Geometry: final body of the model. Coordinates: model frame, mm. A direction names the side the tool comes from. Give positions to 0.01 mm unless a question says otherwise; leave off trailing zeros. Write each loop counter-clockwise with the first axis right and the second up, starting at its lowest first coordinate (ties: lowest second). Pieces come first, ordered by that corner, then holes. Notation, with made-up numbers: (-19, 59.25) -> (-13, 59.25) arc R5 cw to (-13, 68.25) -> close; hole circle Ø5 at (-29.5, -3.5). An arc over 180 degrees is marked (long way). Use CSV: the item, a comma, the result in double quotes. Start each with the question number.
1) Section C-C (y = 15). Output: boundary loops of the cut face in (x, z), plus the area to 3 significant figures.
2) Material intervals for line 1 (X direction, y = -16.5, z = 51.5); line 2 (Y direction, x = 0, z = -2.3); line 3 (Y direction, x = -10, z = -1), sorted ascending. Write a range as [from, to].
3) Set-up query: faces 1 (the face through (-1, 0, 0)), 2 (the face through (74.3, 0, 39)), 3 (the face through (73, 0, 76)). Return all of +Z, -Z, +X, -X, +Y, -Y with unobstructed straight access to the full face (end or side cutting, diameter ignored); none if empty.
4) Section B-B (z = 74.5). Output: boundary loops of the cut face in (x, y), plus the area to 3 significant figures.
5) Section A-A (z = 12.5). Output: boundary loops of the cut face in (x, y).
6) Draft query along Z for faces 4 (the face through (-72.821, -0.93, 85.986)), 5 (the face through (-72.82, 0.07, 54.3)), 6 (the face through (-72.496, 0.28, -1.289)), 7 (the face through (71.3, 0, 39)). Return one class per face: pulls with the +Z half, pulls with the -Z half, needs draft (parallel to the pull), parting line crosses it, or undercut.
7) Contact query for flat-ended pins moving along their axis: P1, Ø12, axis at x = -16.5, y = -18.5, coming from the +Z side; P2, Ø4.5, axis at y = -15, z = 74.5, coming from the +X side. Output: stop coordinate, or through.
8) Section D-D (x = -61.5). Output: boundary loops of the cut face in (y, z), plus the area to 3 significant figures.
```python
from build123d import *

# Parameters (mm, degrees)
ESQUISSE1_W                           = 142.6
ESQUISSE1_H                           = 40
T_LE_DE_BASE_PLI_E1_DEPTH             = 3
T_LE_PLI_E_SUR_AR_TE1_STRIP_W         = 18
T_LE_PLI_E_SUR_AR_TE1_STRIP_H         = 3
T_LE_PLI_E_SUR_AR_TE1_STRIP_CUT_DEPTH = 40
T_LE_PLI_E_SUR_AR_TE1_DEPTH           = 40
T_LE_PLI_E_SUR_AR_TE2_STRIP_W         = 18
T_LE_PLI_E_SUR_AR_TE2_STRIP_H         = 3
T_LE_PLI_E_SUR_AR_TE2_STRIP_CUT_DEPTH = 40
T_LE_PLI_E_SUR_AR_TE2_DEPTH           = 40
ENL_V_MAT_EXTRU_1_REACH               = 97.166
ESQUISSE14_R                          = 1.25
PATTE1_DEPTH                          = 3
ENL_V_MAT_EXTRU_2_REACH               = 170.101
ESQUISSE19_R                          = 1.25
PATTE2_START                          = -3
PATTE2_DEPTH                          = 3
ENL_V_MAT_EXTRU_3_REACH               = 170.101
ESQUISSE24_R                          = 1.7
ESQUISSE25_R                          = 30
ESQUISSE25_R_2                        = 1.65
ESQUISSE25_R_3                        = 1.7
BOSS_EXTRU_1_DEPTH                    = 3
CONG_1_R                              = 20


# Sheet-metal steps are written as plain solids
with BuildPart() as part:
    # Esquisse1 → Tôle de base pliée1 (new body)
    with BuildSketch(Plane.XY):
        Rectangle(ESQUISSE1_W, ESQUISSE1_H)
    extrude(amount=-T_LE_DE_BASE_PLI_E1_DEPTH)

    # Tôle pliée sur arête1 strip (across the edge) → Tôle pliée sur arête1 strip cut (cut)
    with BuildSketch(Plane(origin=(-71.3, 20, 0), x_dir=(1, 0, 0), z_dir=(0, -1, 0))):
        with Locations((-6, -1.5)):
            Rectangle(T_LE_PLI_E_SUR_AR_TE1_STRIP_W, T_LE_PLI_E_SUR_AR_TE1_STRIP_H)
    extrude(amount=T_LE_PLI_E_SUR_AR_TE1_STRIP_CUT_DEPTH, mode=Mode.SUBTRACT)

    # Tôle pliée sur arête1 section (across the edge) → Tôle pliée sur arête1 (add)
    with BuildSketch(Plane(origin=(-71.3, 20, 0), x_dir=(1, 0, 0), z_dir=(0, -1, 0))):
        with BuildLine():
            Line((-3, 3), (-3, 56))
            Line((-3, 56), (0, 56))
            Line((0, 56), (0, 3))
            ThreePointArc((0, 3), (0.878679656, 0.878679656), (3, 0))
            Line((3, 0), (3, -3))
            ThreePointArc((3, -3), (-1.242640687, -1.242640687), (-3, 3))
        make_face()
    extrude(amount=T_LE_PLI_E_SUR_AR_TE1_DEPTH)

    # Tôle pliée sur arête2 strip (across the edge) → Tôle pliée sur arête2 strip cut (cut)
    with BuildSketch(Plane(origin=(71.3, -20, 0), x_dir=(-1, 0, 0), z_dir=(0, 1, 0))):
        with Locations((-6, -1.5)):
            Rectangle(T_LE_PLI_E_SUR_AR_TE2_STRIP_W, T_LE_PLI_E_SUR_AR_TE2_STRIP_H)
    extrude(amount=T_LE_PLI_E_SUR_AR_TE2_STRIP_CUT_DEPTH, mode=Mode.SUBTRACT)

    # Tôle pliée sur arête2 section (across the edge) → Tôle pliée sur arête2 (add)
    with BuildSketch(Plane(origin=(71.3, -20, 0), x_dir=(-1, 0, 0), z_dir=(0, 1, 0))):
        with BuildLine():
            Line((-3, 3), (-3, 56))
            Line((-3, 56), (0, 56))
            Line((0, 56), (0, 3))
            ThreePointArc((0, 3), (0.878679656, 0.878679656), (3, 0))
            Line((3, 0), (3, -3))
            ThreePointArc((3, -3), (-1.242640687, -1.242640687), (-3, 3))
        make_face()
    extrude(amount=T_LE_PLI_E_SUR_AR_TE2_DEPTH)

    # Esquisse14 → Enlèv. mat.-Extru.1 (cut, up to next)
    with BuildSketch(Plane.XY, mode=Mode.PRIVATE) as enl_v_mat_extru_1_sk1:
        with Locations((0, 10)):
            Circle(ESQUISSE14_R)
    enl_v_mat_extru_1_tool1 = extrude(enl_v_mat_extru_1_sk1.sketch, amount=-ENL_V_MAT_EXTRU_1_REACH, mode=Mode.PRIVATE) & part.part
    # Esquisse14 → Enlèv. mat.-Extru.1 (cut, up to next)
    with BuildSketch(Plane.XY, mode=Mode.PRIVATE) as enl_v_mat_extru_1_sk2:
        with Locations((10, 0)):
            Circle(ESQUISSE14_R)
    enl_v_mat_extru_1_tool2 = extrude(enl_v_mat_extru_1_sk2.sketch, amount=-ENL_V_MAT_EXTRU_1_REACH, mode=Mode.PRIVATE) & part.part
    # Esquisse14 → Enlèv. mat.-Extru.1 (cut, up to next)
    with BuildSketch(Plane.XY, mode=Mode.PRIVATE) as enl_v_mat_extru_1_sk3:
        with Locations((0, -10)):
            Circle(ESQUISSE14_R)
    enl_v_mat_extru_1_tool3 = extrude(enl_v_mat_extru_1_sk3.sketch, amount=-ENL_V_MAT_EXTRU_1_REACH, mode=Mode.PRIVATE) & part.part
    # Esquisse14 → Enlèv. mat.-Extru.1 (cut, up to next)
    with BuildSketch(Plane.XY, mode=Mode.PRIVATE) as enl_v_mat_extru_1_sk4:
        with Locations((-10, 0)):
            Circle(ESQUISSE14_R)
    enl_v_mat_extru_1_tool4 = extrude(enl_v_mat_extru_1_sk4.sketch, amount=-ENL_V_MAT_EXTRU_1_REACH, mode=Mode.PRIVATE) & part.part
    add(enl_v_mat_extru_1_tool1.solids().sort_by_distance((0, 10, 0))[0], mode=Mode.SUBTRACT)
    add(enl_v_mat_extru_1_tool2.solids().sort_by_distance((10, 0, 0))[0], mode=Mode.SUBTRACT)
    add(enl_v_mat_extru_1_tool3.solids().sort_by_distance((0, -10, 0))[0], mode=Mode.SUBTRACT)
    add(enl_v_mat_extru_1_tool4.solids().sort_by_distance((-10, 0, 0))[0], mode=Mode.SUBTRACT)

    # Esquisse16 → Patte1 (add)
    with BuildSketch(Plane(origin=(74.3, 0, 0), x_dir=(0, 0, -1), z_dir=(1, 0, 0))):
        with BuildLine():
            Line((-56, 20), (-56, -20))
            ThreePointArc((-56, -20), (-76, 0), (-56, 20))
        make_face()
    extrude(amount=-PATTE1_DEPTH)

    # Esquisse19 → Enlèv. mat.-Extru.2 (cut, up to next)
    with BuildSketch(Plane(origin=(74.3, 0, 0), x_dir=(0, 0, -1), z_dir=(1, 0, 0)), mode=Mode.PRIVATE) as enl_v_mat_extru_2_sk1:
        with Locations((-64.838834765, 8.838834765)):
            Circle(ESQUISSE19_R)
    enl_v_mat_extru_2_tool1 = extrude(enl_v_mat_extru_2_sk1.sketch, amount=-ENL_V_MAT_EXTRU_2_REACH, mode=Mode.PRIVATE) & part.part
    # Esquisse19 → Enlèv. mat.-Extru.2 (cut, up to next)
    with BuildSketch(Plane(origin=(74.3, 0, 0), x_dir=(0, 0, -1), z_dir=(1, 0, 0)), mode=Mode.PRIVATE) as enl_v_mat_extru_2_sk2:
        with Locations((-47.161165235, 8.838834765)):
            Circle(ESQUISSE19_R)
    enl_v_mat_extru_2_tool2 = extrude(enl_v_mat_extru_2_sk2.sketch, amount=-ENL_V_MAT_EXTRU_2_REACH, mode=Mode.PRIVATE) & part.part
    # Esquisse19 → Enlèv. mat.-Extru.2 (cut, up to next)
    with BuildSketch(Plane(origin=(74.3, 0, 0), x_dir=(0, 0, -1), z_dir=(1, 0, 0)), mode=Mode.PRIVATE) as enl_v_mat_extru_2_sk3:
        with Locations((-47.161165235, -8.838834765)):
            Circle(ESQUISSE19_R)
    enl_v_mat_extru_2_tool3 = extrude(enl_v_mat_extru_2_sk3.sketch, amount=-ENL_V_MAT_EXTRU_2_REACH, mode=Mode.PRIVATE) & part.part
    # Esquisse19 → Enlèv. mat.-Extru.2 (cut, up to next)
    with BuildSketch(Plane(origin=(74.3, 0, 0), x_dir=(0, 0, -1), z_dir=(1, 0, 0)), mode=Mode.PRIVATE) as enl_v_mat_extru_2_sk4:
        with Locations((-64.838834765, -8.838834765)):
            Circle(ESQUISSE19_R)
    enl_v_mat_extru_2_tool4 = extrude(enl_v_mat_extru_2_sk4.sketch, amount=-ENL_V_MAT_EXTRU_2_REACH, mode=Mode.PRIVATE) & part.part
    add(enl_v_mat_extru_2_tool1.solids().sort_by_distance((74.3, 8.838835, 64.838835))[0], mode=Mode.SUBTRACT)
    add(enl_v_mat_extru_2_tool2.solids().sort_by_distance((74.3, 8.838835, 47.161165))[0], mode=Mode.SUBTRACT)
    add(enl_v_mat_extru_2_tool3.solids().sort_by_distance((74.3, -8.838835, 47.161165))[0], mode=Mode.SUBTRACT)
    add(enl_v_mat_extru_2_tool4.solids().sort_by_distance((74.3, -8.838835, 64.838835))[0], mode=Mode.SUBTRACT)

    # Esquisse20 → Patte2 (add)
    with BuildSketch(Plane.ZY.offset(74.3).offset(PATTE2_START)):
        with BuildLine():
            Line((56, 20), (56, -20))
            ThreePointArc((56, -20), (76, 0), (56, 20))
        make_face()
    extrude(amount=PATTE2_DEPTH)

    # Esquisse24 → Enlèv. mat.-Extru.3 (cut, up to next)
    with BuildSketch(Plane.ZY.offset(74.3), mode=Mode.PRIVATE) as enl_v_mat_extru_3_sk1:
        with Locations((56, 0)):
            Circle(ESQUISSE24_R)
    enl_v_mat_extru_3_tool1 = extrude(enl_v_mat_extru_3_sk1.sketch, amount=-ENL_V_MAT_EXTRU_3_REACH, mode=Mode.PRIVATE) & part.part
    add(enl_v_mat_extru_3_tool1.solids().sort_by_distance((-74.3, 0, 56))[0], mode=Mode.SUBTRACT)

    # Esquisse25 → Boss.-Extru.1 (add)
    with BuildSketch(Plane.ZY.offset(74.3)):
        with Locations((56, 0)):
            Circle(ESQUISSE25_R)
        with Locations((65, 24)):
            Circle(ESQUISSE25_R_2, mode=Mode.SUBTRACT)
        with Locations((74.5, -15)):
            Circle(ESQUISSE25_R_2, mode=Mode.SUBTRACT)
        with Locations((56, 0)):
            Circle(ESQUISSE25_R_3, mode=Mode.SUBTRACT)
    extrude(amount=-BOSS_EXTRU_1_DEPTH)

    # Congé1
    cong_1_edges = [part.edges().sort_by_distance(p)[0] for p in [
        (-72.8, 20, 33.639320225),
        (-72.8, -20, 33.639320225),
    ]]
    fillet(cong_1_edges, radius=CONG_1_R)


solid = part.part
```
Answers follow:
1,outline,"(-74.3, 3) arc R6 ccw to (-68.3, -3) -> (68.3, -3) arc R6 ccw to (74.3, 3) -> (74.3, 69.23) -> (71.3, 69.23) -> (71.3, 3) arc R3 cw to (68.3, 0) -> (-68.3, 0) arc R3 cw to (-71.3, 3) -> (-71.3, 81.98) -> (-74.3, 81.98) -> close"
1,area,"888 mm^2"
2,line 1,"x = [-74.3, -71.3], [71.3, 74.3]"
2,line 2,"y = [-20, -11.25], [-8.75, 8.75], [11.25, 20]"
2,line 3,"y = [-20, -1.25], [1.25, 20]"
3,face 1,"+Z, +Y, -Y"
3,face 2,"+Z, -Z, +X, +Y, -Y"
3,face 3,"+Z, +X"
4,outline,"(-74.3, -23.62) -> (-71.3, -23.62) -> (-71.3, -16.65) -> (-74.3, -16.65) -> close; (-74.3, -13.35) -> (-71.3, -13.35) -> (-71.3, 23.62) -> (-74.3, 23.62) -> close; (71.3, -7.6) -> (74.3, -7.6) -> (74.3, 7.6) -> (71.3, 7.6) -> close"
4,area,"177 mm^2"
5,outline,"(-74.3, -20) -> (-71.3, -20) -> (-71.3, 20) -> (-74.3, 20) -> close; (71.3, -20) -> (74.3, -20) -> (74.3, 20) -> (71.3, 20) -> close"
6,face 4,"parting line crosses it"
6,face 5,"undercut"
6,face 6,"pulls with the -Z half"
6,face 7,"needs draft"
7,P1,"stops at z = 0"
7,P2,"stops at x = -71.3"
8,outline,"(-20, -3) -> (20, -3) -> (20, 0) -> (-20, 0) -> close"
8,area,"120 mm^2"
